Check sheet for the drawn part. Datum: minimum x, y, z corner. Units: mm. Coordinates: 2 decimals unless noted, no trailing zeros. Loops run counter-clockwise (first coordinate to the right, second up) from the corner with the lowest first, then second, coordinate; pieces in that order, holes last.
Q1. Sectioned sample at A-A (x = 63.5). Enter the section's corners in (y, z).
Q2. Mould release check, pull along Z, two halves, no side actions. Record for the marked faces 1, 2 and 3: +Z half, -Z half, draft (parallel to the pull), parting line (faces both ways), or undercut.
Q3. Material ranges on probe 1 along Z at (x, y) = (63, 11); probe 2 along Z at (x, y) = (96, 63.5); probe 3 along X at (y, z) = (16.25, 63.5), recorded low to high.
Q4. Sectioned sample at C-C (y = 90). Enter the section's corners in (x, z).
Q5. Sectioned sample at D-D (x = 29). Enter the section's corners in (y, z), then the cut area to 3 significant figures.
Q6. Go/stop test with a flat-tipped pin: P1, Ø2, axis at x = 61, z = 83, coming from the -Y side. Record where the tip stops, or that it passes through.
Q7. Sectioned sample at B-B (z = 63.5). Enter the section's corners in (x, y), then the cut area to 3 significant figures.
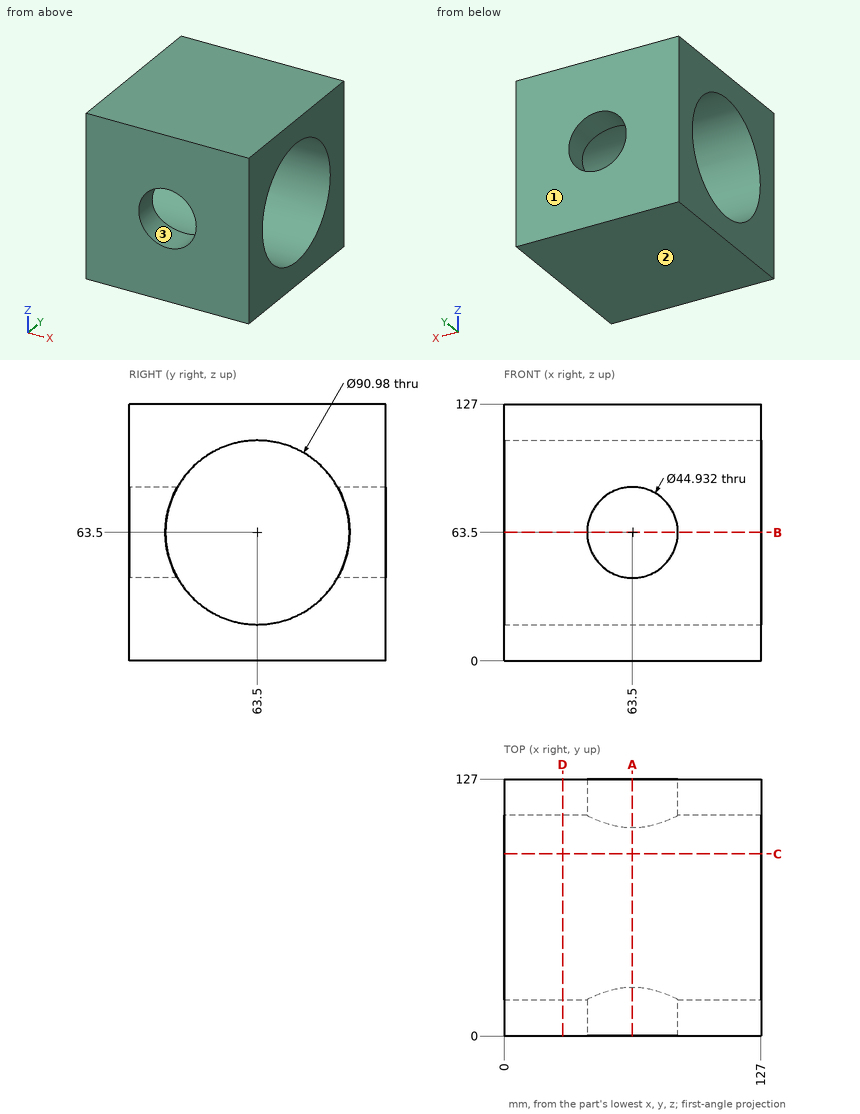
Geometry check:
1. outline: (0, 0) - (127, 0) - (127, 41.03) - (103.06, 41.03) arc R45.49 cw to (23.94, 41.03) - (0, 41.03) - close; (0, 85.97) - (23.94, 85.97) arc R45.49 cw to (103.06, 85.97) - (127, 85.97) - (127, 127) - (0, 127) - close
2. face 1: draft
2. face 2: -Z half
2. face 3: undercut
3. probe 1: z = 0 to 41.04, 85.96 to 127
3. probe 2: z = 0 to 18.01, 108.99 to 127
3. probe 3: x = 0 to 41.03, 85.97 to 127
4. outline: (0, 0) - (127, 0) - (127, 26.53) - (0, 26.53) - close; (0, 100.47) - (127, 100.47) - (127, 127) - (0, 127) - close
5. outline: (0, 0) - (127, 0) - (127, 127) - (0, 127) - close; hole circle Ø90.98 at (63.5, 63.5)
5. area: 9,630 mm2
6. P1: passes through
7. outline: (0, 0) - (41.03, 0) - (41.03, 18.01) - (0, 18.01) - close; (0, 108.99) - (41.03, 108.99) - (41.03, 127) - (0, 127) - close; (85.97, 0) - (127, 0) - (127, 18.01) - (85.97, 18.01) - close; (85.97, 108.99) - (127, 108.99) - (127, 127) - (85.97, 127) - close
7. area: 2,960 mm2
